Check sheet for the drawn part. Datum: minimum x, y, z corner. Units: mm. A direction names the side the tool comes from. Give positions to 0.01 mm unless a question says otherwise; leave off trailing zeros. Write each loop counter-clockwise with the first axis right and the second up, starting at its lowest first coordinate (ties: lowest second). Pieces come first, ordered by that corner, then holes.
(1) Cross-section at B-B (y = 72). Record the boundary of the cut face in (x, z), and give its area (3 significant figures).
(2) Cross-section at A-A (z = 115.5). Record the boundary of the cut face in (x, y).
(3) Cross-section at C-C (x = 185). Record the boundary of the cut face in (y, z).
(4) Thickness scan on line 1 along X through (y, z) = (55, 36.5); line 2 along X through (y, z) = (207, 100); line 3 along Y through (x, z) = (68.5, 49). Record the ranges inside material, lowest first.
(5) Cross-section at D-D (z = 188.5). Record the boundary of the cut face in (x, y), and give its area (3 significant figures).
(6) Tool access check on the marked faces 1 and 2. Record the directions out of +Z, -Z, +X, -X, +Y, -Y that give a thin tool (end or side, any length) a straight path to the whole face; none if there is none.
(7) Depth check by flat-ended pin: P1, Ø5, axis at x = 215.5, z = 141.5, coming from the -Y side. Enter the tip coordinate at first touch or a pass-through.
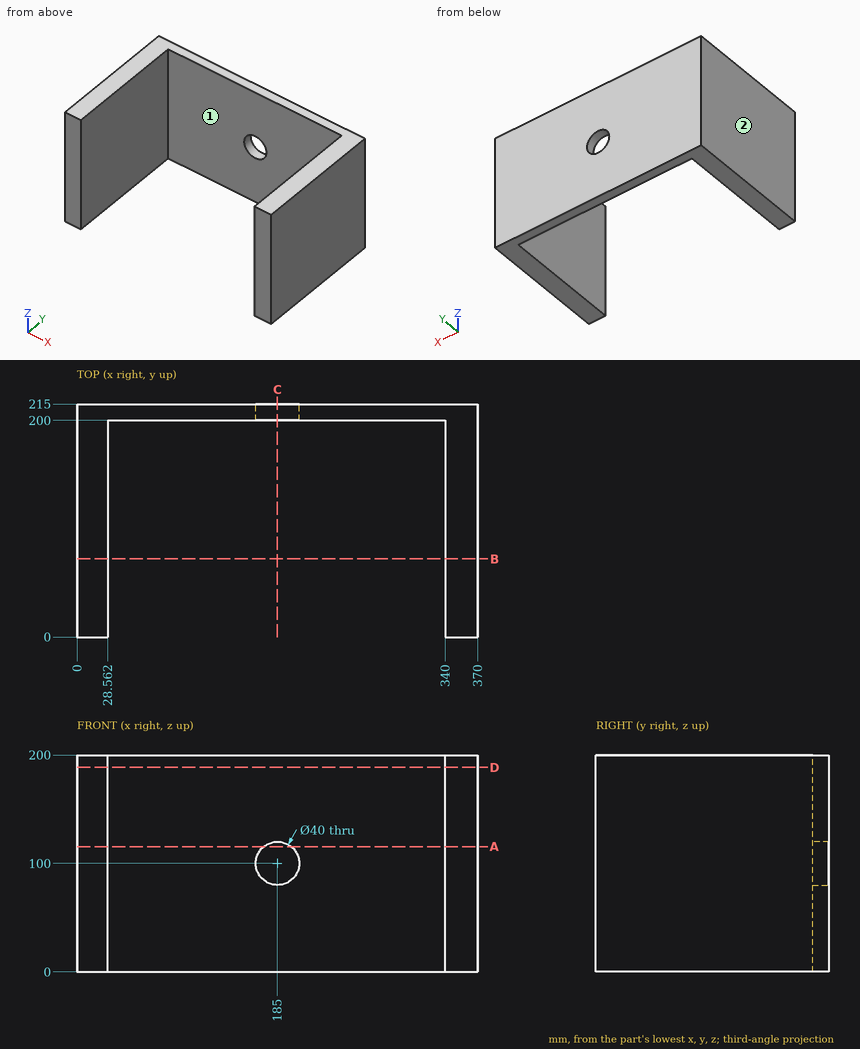
Reply:
1. outline: (0, 0) - (28.56, 0) - (28.56, 200) - (0, 200) - close; (340, 0) - (370, 0) - (370, 200) - (340, 200) - close
1. area: 11,700 mm2
2. outline: (0, 0) - (28.56, 0) - (28.56, 200) - (172.36, 200) - (172.36, 215) - (0, 215) - close; (197.64, 200) - (340, 200) - (340, 0) - (370, 0) - (370, 215) - (197.64, 215) - close
3. outline: (200, 0) - (215, 0) - (215, 80) - (200, 80) - close; (200, 120) - (215, 120) - (215, 200) - (200, 200) - close
4. line 1: x = 0 to 28.56, 340 to 370
4. line 2: x = 0 to 165, 205 to 370
4. line 3: y = 200 to 215
5. outline: (0, 0) - (28.56, 0) - (28.56, 200) - (340, 200) - (340, 0) - (370, 0) - (370, 215) - (0, 215) - close
5. area: 17,300 mm2
6. face 1: +Z, -Z, -Y
6. face 2: +Z, -Z, -X, +Y, -Y
7. P1: stops at y = 200
